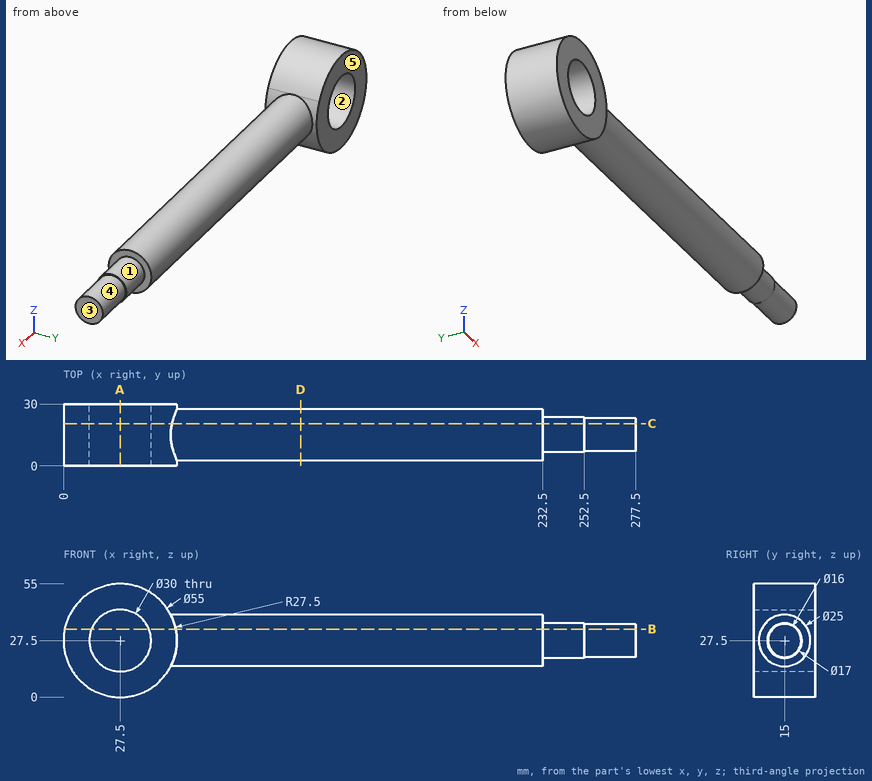
Check sheet for the drawn part. Datum: minimum x, y, z corner. Units: mm. A direction names the side the tool comes from. Round coordinates to 2 decimals unless told otherwise and drop trailing zeros. Order: outer loops, then holes, each group sorted by start corner. A loop starts at its lowest first (then second) coordinate and runs counter-clockwise, first axis right, second up. Notation, with made-up numbers: (80, 35) -> (114, 35) arc R11 ccw to (114, 49) -> close; hole circle Ø9 at (-22, 86). An arc over 180 degrees is marked (long way). Put each result on its own line as item: value.
1) Mould release check, pull along X, two halves, no side actions. Record for the marked faces 1, 2 and 3: +X half, -X half, draft (parallel to the pull), parting line (faces both ways), or undercut.
Final values:
face 1: draft
face 2: undercut
face 3: +X half
2) Depth check by flat-ended pin: pin 1 (4 mm diameter, centred on x = 29, y = 23, fed in from -Z); pin 2 (6 mm diameter, centred on y = 6, z = 35.5, fed in from -X); pin 3 (2 mm diameter, centred on x = 84, y = 15.5, fed in from -Z); pin 4 (12 mm diameter, centred on x = 54, z = 14.5, fed in from +Y). Enter the tip coordinate at first touch or a pass-through.
Final values:
pin 1: stops at z = 0
pin 2: stops at x = 0.46
pin 3: stops at z = 15
pin 4: stops at y = 30
3) Material ranges on line 1 (Z direction, x = 27.5, y = 18.75); line 2 (X direction, y = 9, z = 27); line 3 (X direction, y = 18, z = 41), recorded low to high.
Final values:
line 1: z = 0 to 12.5, 42.5 to 55
line 2: x = 0 to 12.51, 42.49 to 277.5
line 3: x = 3.54 to 20.96, 34.04 to 51.46
4) Section check B-B (z = 33). Record the cut outline in (x, y) (1 decimal), then the cut area to 3 significant figures.
Final values:
outline: (0.6, 0) -> (13.5, 0) -> (13.5, 30) -> (0.6, 30) -> close; (41.5, 0) -> (54.4, 0) -> (54.4, 3.8) -> (232.5, 3.8) -> (232.5, 8.5) -> (252.5, 8.5) -> (252.5, 9.2) -> (277.5, 9.2) -> (277.5, 20.8) -> (252.5, 20.8) -> (252.5, 21.5) -> (232.5, 21.5) -> (232.5, 26.2) -> (54.4, 26.2) -> (54.4, 30) -> (41.5, 30) -> close
area: 5,330 mm^2
5) Section check A-A (x = 27.5). Record the cut outline in (y, z).
Final values:
outline: (0, 0) -> (30, 0) -> (30, 12.5) -> (0, 12.5) -> close; (0, 42.5) -> (30, 42.5) -> (30, 55) -> (0, 55) -> close
6) Section check C-C (y = 20.5). Record the cut outline in (x, z) (1 decimal), then the cut area to 3 significant figures.
Final values:
outline: (52, 40) arc R27.5 ccw (long way) to (52.6, 16.3) -> (232.5, 16.3) -> (232.5, 21) -> (252.5, 21) -> (252.5, 21.7) -> (277.5, 21.7) -> (277.5, 33.3) -> (252.5, 33.3) -> (252.5, 34) -> (232.5, 34) -> (232.5, 38.7) -> (52.6, 38.7) arc R27.5 ccw to start; hole circle Ø30 at (27.5, 27.5)
area: 6,220 mm^2
7) Set-up check for the marked faces 4 and 5: record each of +Z, -Z, +X, -X, +Y, -Y from which the full face is reachable in a straight line by a thin tool's end or side.
Final values:
face 4: +X
face 5: +Z, -Z, +X, -X, +Y
8) Section check D-D (x = 115). Record the cut outline in (y, z), then the cut area to 3 significant figures.
Final values:
outline: circle Ø25 at (15, 27.5)
area: 491 mm^2
